Here's how the part is built. I have some questions about the finished solid (model axes, mm). A direction names the side the tool comes from. Coordinates: 2 decimals unless noted, no trailing zeros. Write each loop counter-clockwise with the first axis right and the second up, starting at its lowest first coordinate (ties: lowest second). Pieces come first, ordered by that corner, then holes.
from build123d import *
from build123d.topology import SkipClean

# Parameters (mm, degrees)
SKETCH2_R              = 9.5
BOSS_EXTRUDE1_DEPTH    = 21
SKETCH3_R              = 4.25
BOSS_EXTRUDE2_DEPTH    = 5
BOSS_EXTRUDE3_START    = 10
SKETCH4_R              = 9.5
BOSS_EXTRUDE3_DEPTH    = 10
CUT_EXTRUDE1_START     = -7.5
CUT_EXTRUDE1_OUTLINE_R = 9.5
CUT_EXTRUDE1_DEPTH     = 7.5
SKETCH6_R              = 9.5
BOSS_EXTRUDE4_DEPTH    = 3


# Read off the part's stored shape, not the designer's step: Cut-Extrude1
with BuildPart() as part:
    # Sketch2 → Boss-Extrude1 (new body)
    with BuildSketch(Plane.XY):
        Circle(SKETCH2_R)
        Polygon((-6.5, -3.75277675), (0, -7.505553499), (6.5, -3.75277675), (6.5, 3.75277675), (0, 7.505553499), (-6.5, 3.75277675), align=None, mode=Mode.SUBTRACT)
    extrude(amount=-BOSS_EXTRUDE1_DEPTH)

    # Sketch3 → Boss-Extrude2 (add)
    with BuildSketch(Plane.XY):
        Polygon((-6.5, -3.75277675), (0, -7.505553499), (6.5, -3.75277675), (6.5, 3.75277675), (0, 7.505553499), (-6.5, 3.75277675), align=None)
        Circle(SKETCH3_R, mode=Mode.SUBTRACT)
    extrude(amount=-BOSS_EXTRUDE2_DEPTH)

    # Sketch4 → Boss-Extrude3 (add)
    with BuildSketch(Plane.XY.offset(BOSS_EXTRUDE3_START)):
        with Locations(Location((0, 0, 0), (0, 0, 270))):
            Circle(SKETCH4_R)
        with BuildLine():
            ThreePointArc((3.929134765, -1.62), (-4.25, 0), (3.929134765, 1.62))
            Line((3.929134765, 1.62), (5.52, 1.62))
            Line((5.52, 1.62), (5.52, -1.62))
            Line((5.52, -1.62), (3.929134765, -1.62))
        make_face(mode=Mode.SUBTRACT)
    extrude(amount=-BOSS_EXTRUDE3_DEPTH)

    # Cut-Extrude1 outline → Cut-Extrude1 (cut)
    with BuildSketch(Plane(origin=(0, 0, -21), x_dir=(-1, 0, 0), z_dir=(0, 0, -1)).offset(CUT_EXTRUDE1_START)):
        Circle(CUT_EXTRUDE1_OUTLINE_R)
        Polygon((6.5, 3.75277675), (6.5, -3.75277675), (0, -7.505553499), (-6.5, -3.75277675), (-6.5, 3.75277675), (0, 7.505553499), align=None, mode=Mode.SUBTRACT)
    extrude(amount=CUT_EXTRUDE1_DEPTH, mode=Mode.SUBTRACT)

    # Sketch6 → Boss-Extrude4 (add)
    with SkipClean():  # the faces are left unmerged after this step: merging them gives an invalid solid
        with BuildSketch(Plane(origin=(0, 0, -13.5), x_dir=(-1, 0, 0), z_dir=(0, 0, -1))):
            with Locations(Location((0, 0, 0), (0, 0, 270))):
                Circle(SKETCH6_R)
            Polygon((6.5, 3.75277675), (6.5, -3.75277675), (0, -7.505553499), (-6.5, -3.75277675), (-6.5, 3.75277675), (0, 7.505553499), align=None, mode=Mode.SUBTRACT)
        extrude(amount=BOSS_EXTRUDE4_DEPTH)
    add(part.part.scale(1), mode=Mode.REPLACE)  # the faces are merged on a copy


solid = part.part
1. I want a section at B-B (z = -9.25). List the corners of the cut face in (x, y) for me, then the cut area to 3 significant figures.
2. For pin 1 Ø5 at (y, z) = (7, -2.5) entering from -X; pin 2 Ø1.5 at (y, z) = (2, -15) entering from +X; pin 3 Ø11 at (x, y) = (0, 0) entering from -Z, each with a flat end and sliding along its axis, tell me the tip position at first contact or that it passes through.
3. If I drill on line 1 (Y direction, x = 0, z = -3.4); line 2 (Z direction, x = -5, y = 2.5); line 3 (Y direction, x = 4.5, z = 7.75), over which ranges is the centre line in solid material (lowest first)?
4. I want a section at C-C (x = 0.75). List the corners of the cut face in (y, z) for me, then the cut area to 3 significant figures.
5. On a 3-axis mill with a long thin cutter (end or side, diameter ignored), from which of +Z, -Z, +X, -X, +Y, -Y can I reach the whole of each face in a straight line? I mean faces 1 (the face through (-2.2, 6.5, -16.5)), 2 (the face through (5, 1.62, 5)). Say none if no direction works.
6. I want a section at A-A (y = 0). List the corners of the cut face in (x, z) for me.
7. I want a section at D-D (x = 4.75). List the corners of the cut face in (y, z) for me, then the cut area to 3 significant figures.
8. Thinking about a two-plate mould opening in Y: for faces 3 (the face through (-4.4, 0.1, -5)), 4 (the face through (-4, -2, 10)), which applies, pulls with the +Y half, pulls with the -Y half, needs draft (parallel to the pull), parting line crosses it, or undercut?
Response values:
1. outline: circle Ø19 at (0, 0); hole (-6.5, -3.75) - (0, -7.51) - (6.5, -3.75) - (6.5, 3.75) - (0, 7.51) - (-6.5, 3.75) - close
1. area: 137 mm2
2. pin 1: stops at x = -8.37
2. pin 2: stops at x = 9.42
2. pin 3: stops at z = -5
3. line 1: y = -9.5 to -4.25, 4.25 to 9.5
3. line 2: z = -5 to 10
3. line 3: y = -8.37 to -1.62, 1.62 to 8.37
4. outline: (-9.47, -16.5) - (-7.07, -16.5) - (-7.07, -5) - (-4.18, -5) - (-4.18, 10) - (-9.47, 10) - close; (4.18, -5) - (7.07, -5) - (7.07, -16.5) - (9.47, -16.5) - (9.47, 10) - (4.18, 10) - close
4. area: 214 mm2
5. face 1: -Z, +X, -X, +Y, -Y
5. face 2: +Z
6. outline: (-9.5, -16.5) - (-6.5, -16.5) - (-6.5, -5) - (-4.25, -5) - (-4.25, 10) - (-9.5, 10) - close; (4.25, -5) - (6.5, -5) - (6.5, -16.5) - (9.5, -16.5) - (9.5, 10) - (5.52, 10) - (5.52, 0) - (4.25, 0) - close
7. outline: (-8.23, -16.5) - (-4.76, -16.5) - (-4.76, -5) - (4.76, -5) - (4.76, -16.5) - (8.23, -16.5) - (8.23, 10) - (1.62, 10) - (1.62, 0) - (-1.62, 0) - (-1.62, 10) - (-8.23, 10) - close
7. area: 294 mm2
8. face 3: undercut
8. face 4: needs draft
